```python
from build123d import *

# Parameters (mm, degrees)
F0_W     = 76.2
F0_H     = 47.625
F1_DEPTH = 3.175
F2_W     = 76.2
F2_H     = 47.625
F2_W_2   = 69.85
F2_H_2   = 1.5875
F3_DEPTH = 139.7
F4_W     = 3.175
F4_H     = 3.175
F5_DEPTH = 47.625
F6_DEPTH = 2540


with BuildPart() as f1:
    # F0 (on Front) → F1 (new body)
    with BuildSketch(Plane.XZ):
        with Locations((38.1, 23.8125)):
            Rectangle(F0_W, F0_H)
    extrude(amount=F1_DEPTH)

    # F2 (on face) → F3 (join)
    with BuildSketch(Plane.XZ.offset(3.175)):
        with Locations((38.1, 23.8125)):
            Rectangle(F2_W, F2_H)
        Polygon((73.025, 3.175), (3.175, 3.175), (3.175, 22.225), (3.175, 23.8125), (3.175, 25.4), (3.175, 32.016575672), (3.175, 44.45), (73.025, 44.45), (73.025, 32.016575672), (73.025, 25.4), (73.025, 23.8125), (73.025, 22.225), align=None, mode=Mode.SUBTRACT)
        with Locations((38.1, 23.01875)):
            Rectangle(F2_W_2, F2_H_2)
        with Locations((38.1, 24.60625)):
            Rectangle(F2_W_2, F2_H_2)
    extrude(amount=F3_DEPTH)

    # F4 (on face) → F5 (join, through all)
    with BuildSketch(Plane.XY.offset(47.625)):
        with BuildLine():
            Line((41.275, -149.225), (38.1, -149.225))
            Line((38.1, -149.225), (34.925, -149.225))
            ThreePointArc((34.925, -149.225), (33.9950640303, -151.4700640303), (31.75, -152.4))
            Line((31.75, -152.4), (44.45, -152.4))
            ThreePointArc((44.45, -152.4), (42.2049359697, -151.4700640303), (41.275, -149.225))
        make_face()
        with BuildLine():
            ThreePointArc((31.75, -152.4), (33.9950640303, -151.4700640303), (34.925, -149.225))
            Line((34.925, -149.225), (31.75, -149.225))
            Line((31.75, -149.225), (31.75, -152.4))
        make_face()
        with BuildLine():
            Line((31.75, -149.225), (34.925, -149.225))
            ThreePointArc((34.925, -149.225), (33.9950640303, -146.9799359697), (31.75, -146.05))
            ThreePointArc((31.75, -146.05), (28.575, -149.225), (31.75, -152.4))
            Line((31.75, -152.4), (31.75, -149.225))
        make_face()
        with BuildLine():
            Line((38.1, -149.225), (38.1, -146.05))
            Line((38.1, -146.05), (34.925, -146.05))
            Line((34.925, -146.05), (31.75, -146.05))
            ThreePointArc((31.75, -146.05), (33.9950640303, -146.9799359697), (34.925, -149.225))
            Line((34.925, -149.225), (38.1, -149.225))
        make_face()
        with BuildLine():
            Line((41.275, -146.05), (38.1, -146.05))
            Line((38.1, -146.05), (38.1, -149.225))
            Line((38.1, -149.225), (41.275, -149.225))
            ThreePointArc((41.275, -149.225), (42.2049359697, -146.9799359697), (44.45, -146.05))
            Line((44.45, -146.05), (41.275, -146.05))
        make_face()
        with BuildLine():
            ThreePointArc((47.625, -149.225), (46.6950640303, -146.9799359697), (44.45, -146.05))
            Line((44.45, -146.05), (44.45, -149.225))
            Line((44.45, -149.225), (44.45, -152.4))
            ThreePointArc((44.45, -152.4), (46.6950640303, -151.4700640303), (47.625, -149.225))
        make_face()
        with BuildLine():
            ThreePointArc((44.45, -146.05), (42.2049359697, -146.9799359697), (41.275, -149.225))
            Line((41.275, -149.225), (44.45, -149.225))
            Line((44.45, -149.225), (44.45, -146.05))
        make_face()
        with BuildLine():
            Line((44.45, -149.225), (41.275, -149.225))
            ThreePointArc((41.275, -149.225), (42.2049359697, -151.4700640303), (44.45, -152.4))
            Line((44.45, -152.4), (44.45, -149.225))
        make_face()
        with Locations((39.6875, -144.4625)):
            Rectangle(F4_W, F4_H)
        with Locations((36.5125, -144.4625)):
            Rectangle(F4_W, F4_H)
    extrude(amount=-F5_DEPTH)

    # F6 (cut): faces of the model
    f6_faces = [f1.faces().sort_by_distance(p)[0] for p in [
        (38.1, -3.175, 12.7),
        (38.1, -3.175, 34.925),
    ]]
    extrude(f6_faces, amount=F6_DEPTH, mode=Mode.SUBTRACT)


solid = f1.part
```
Source: CAD feature listing. Evaluate the final solid. Frame: model axes, mm. A direction names the side the tool comes from. Give positions to 0.01 mm unless a question says otherwise; leave off trailing zeros. Loops run counter-clockwise (first coordinate to the right, second up) from the corner with the lowest first, then second, coordinate; pieces in that order, holes last. Notation, with made-up numbers: (74.25, 9) -> (116.25, 9) arc R14 cw to (116.25, 16) -> close; hole circle Ø8 at (6, 63). An arc over 180 degrees is marked (long way). Put each result on its own line as item: value. Start each with the question number.
1) Reachability of faces 5 (the face through (41.275, -144, 46)), 6 (the face through (33, -146.05, 2)), 7 (the face through (38, -75, 0)), 8 (the face through (38, -3.175, 13)) from +Z, -Z, +X, -X, +Y, -Y: full face, straight path, thin tool, end or side. Return the list, or none.
2) Cut plane C-C (y = -85). Return loops of the section in (x, z) (3 decimals).
3) Contact query for flat-ended pins moving along their axis: P1, Ø1.6, axis at y = -144.5, z = 45.5, coming from the +X side (3 decimals); P2, Ø8, axis at x = 50.5, z = 30.5, coming from the -Y side (3 decimals). Output: stop coordinate, or through.
4) Cut plane A-A (z = 18). Return loops of the section in (x, y) (3 decimals).
5) Draft query along X for faces 1 (the face through (34.925, -144, 24)), 2 (the face through (38, -77, 25.4)), 3 (the face through (38, -75, 47.625)), 4 (the face through (41.275, -144, 2)). Return one class per face: released by +X, released by -X, zero draft, split by the parting line, or undercut.
6) Cut plane B-B (x = 24). Return loops of the section in (y, z) (3 decimals), then the cut area to 3 significant figures.
7) Material intervals for probe 1 along Z at (x, y) = (53.5, -83.5) (3 decimals); probe 2 along X at (y, z) = (-67, 37) (3 decimals); probe 3 along Y at (x, z) = (13, 17) (3 decimals), sorted ascending.
Results are:
1. face 5: +Z, -Z, +X
1. face 6: +Z, -Z, -X
1. face 7: -Z, +X, -X, +Y, -Y
1. face 8: -Y
2. outline: (0, 0) -> (76.2, 0) -> (76.2, 47.625) -> (0, 47.625) -> close; hole (3.175, 3.175) -> (73.025, 3.175) -> (73.025, 22.225) -> (3.175, 22.225) -> close; hole (3.175, 25.4) -> (73.025, 25.4) -> (73.025, 44.45) -> (3.175, 44.45) -> close
3. P1: stops at x = 41.275
3. P2: stops at y = -3.175
4. outline: (0, -142.875) -> (3.175, -142.875) -> (3.175, -3.175) -> (73.025, -3.175) -> (73.025, -142.875) -> (76.2, -142.875) -> (76.2, 0) -> (0, 0) -> close
5. face 1: released by -X
5. face 2: undercut
5. face 3: zero draft
5. face 4: released by +X
6. outline: (-142.875, 0) -> (0, 0) -> (0, 47.625) -> (-142.875, 47.625) -> (-142.875, 44.45) -> (-3.175, 44.45) -> (-3.175, 25.4) -> (-142.875, 25.4) -> (-142.875, 22.225) -> (-3.175, 22.225) -> (-3.175, 3.175) -> (-142.875, 3.175) -> close
6. area: 1,480 mm2
7. probe 1: z = 0 to 3.175, 22.225 to 25.4, 44.45 to 47.625
7. probe 2: x = 0 to 3.175, 73.025 to 76.2
7. probe 3: y = -3.175 to 0
